```python
from build123d import *

# Parameters (mm, degrees)
CROQUIS2_R            = 43
CORTAR_EXTRUIR1_DEPTH = 2
CROQUIS4_R            = 40
CORTAR_EXTRUIR2_DEPTH = 3
CROQUIS6_R            = 30
CORTAR_EXTRUIR3_DEPTH = 8.5
CROQUIS8_R            = 30
CORTAR_EXTRUIR4_DEPTH = 1
CROQUIS9_R            = 25
CORTAR_EXTRUIR5_DEPTH = 1.5
CROQUIS10_R           = 15
CORTAR_EXTRUIR6_DEPTH = 13
CROQUIS11_R           = 12.5
CORTAR_EXTRUIR7_DEPTH = 18.5
CROQUIS12_R           = 9
CORTAR_EXTRUIR8_DEPTH = 22.5


with BuildPart() as part:
    # Croquis1 → Revolución1 (revolve)
    with BuildSketch(Plane.XY):
        Polygon((0, 0), (60, 0), (60, 12), (43, 12), (30, 27), (30, 35), (0, 35), align=None)
    revolve(axis=Axis((0, 35, 0), (0, -1, 0)))

    # Croquis2 → Cortar-Extruir1 (cut)
    with BuildSketch(Plane.XZ):
        Circle(CROQUIS2_R)
    extrude(amount=-CORTAR_EXTRUIR1_DEPTH, mode=Mode.SUBTRACT)

    # Croquis4 → Cortar-Extruir2 (cut)
    with BuildSketch(Plane.XZ.offset(-2)):
        Circle(CROQUIS4_R)
    extrude(amount=-CORTAR_EXTRUIR2_DEPTH, mode=Mode.SUBTRACT)

    # Croquis5 → Revolución2 (revolve)
    with BuildSketch(Plane.XY):
        Polygon((-40, 2), (-43, 0), (-43, 2), align=None)
    revolve(axis=Axis((0, 0, 0), (0, 1, 0)))

    # Croquis6 → Cortar-Extruir3 (cut)
    with BuildSketch(Plane.XZ.offset(-5)):
        Circle(CROQUIS6_R)
    extrude(amount=-CORTAR_EXTRUIR3_DEPTH, mode=Mode.SUBTRACT)

    # Croquis7 → Cortar-Revolución1 (revolve, cut)
    with BuildSketch(Plane.XY):
        Polygon((-40, 5), (-30, 5), (-30, 13.5), align=None)
    revolve(axis=Axis((0, 0, 0), (0, 1, 0)), mode=Mode.SUBTRACT)

    # Croquis8 → Cortar-Extruir4 (cut)
    with BuildSketch(Plane.XZ.offset(-13.5)):
        Circle(CROQUIS8_R)
    extrude(amount=-CORTAR_EXTRUIR4_DEPTH, mode=Mode.SUBTRACT)

    # Croquis9 → Cortar-Extruir5 (cut)
    with BuildSketch(Plane(origin=(0, 35, 0), x_dir=(1, 0, 0), z_dir=(0, 1, 0))):
        Circle(CROQUIS9_R)
    extrude(amount=-CORTAR_EXTRUIR5_DEPTH, mode=Mode.SUBTRACT)

    # Croquis10 → Cortar-Extruir6 (cut)
    with BuildSketch(Plane(origin=(0, 33.5, 0), x_dir=(1, 0, 0), z_dir=(0, 1, 0))):
        Circle(CROQUIS10_R)
    extrude(amount=-CORTAR_EXTRUIR6_DEPTH, mode=Mode.SUBTRACT)

    # Croquis11 → Cortar-Extruir7 (cut)
    with BuildSketch(Plane(origin=(0, 35, 0), x_dir=(1, 0, 0), z_dir=(0, 1, 0))):
        Circle(CROQUIS11_R)
    extrude(amount=-CORTAR_EXTRUIR7_DEPTH, mode=Mode.SUBTRACT)

    # Croquis12 → Cortar-Extruir8 (cut)
    with BuildSketch(Plane(origin=(0, 35, 0), x_dir=(1, 0, 0), z_dir=(0, 1, 0))):
        Circle(CROQUIS12_R)
    extrude(amount=-CORTAR_EXTRUIR8_DEPTH, mode=Mode.SUBTRACT)


solid = part.part
```
Verification items for the finished model (mm, model axes). A direction names the side the tool comes from. Round coordinates to 2 decimals unless told otherwise and drop trailing zeros. Write each loop counter-clockwise with the first axis right and the second up, starting at its lowest first coordinate (ties: lowest second). Pieces come first, ordered by that corner, then holes. Notation, with made-up numbers: (75.5, 22) - (94.5, 22) arc R17 cw to (94.5, 39) - close; hole circle Ø3 at (-26, 83.5). An arc over 180 degrees is marked (long way). Answer as a JSON object with one key per item and string values. Group by question number.
Q1. Tool access check on faces 4 (the cylindrical face through (-8.67, 3.48, -39.05)), 5 (the cylindrical face through (-1.172, 15.514, -8.923)), 6 (the cylindrical face through (-29.97, 31.06, 1.32)). Record the directions out of +Z, -Z, +X, -X, +Y, -Y that give a thin tool (end or side, any length) a straight path to the whole face; none if there is none.
Q2. Mould release check, pull along X, two halves, no side actions. Record for faces 1 (the flat face through (-14, 12, 41)), 2 (the cylindrical face through (-59.94, 6.08, 2.64)), 3 (the cylindrical face through (23.846, 34.26, -7.509)): released by +X, released by -X, zero draft, split by the parting line, or undercut.
Q3. Thickness scan on line 1 (X direction, y = 15.45, z = 0); line 2 (Z direction, x = 0, y = 2.85); line 3 (Y direction, x = -8.5, z = -13). Record the ranges inside material, lowest first.
Q4. Section check B-B, the plane y = 18.5. Enter the section's corners in (x, z).
Q5. Section check A-A, the plane y = 10. Enter the section's corners in (x, z), plus the area to 3 significant figures.
Q6. Go/stop test with flat-tipped pins: pin 1 Ø4 at (y, z) = (17.5, -5.5) entering from -X; pin 2 Ø4 at (y, z) = (5, 38) entering from -X; pin 3 Ø4 at (x, y) = (7.5, 15) entering from -Z. Record where each tip stops, or that it passes through.
Found:
{
 "1": {"face 4": "-Y", "face 5": "+Y, -Y", "face 6": "+Y"},
 "2": {"face 1": "zero draft", "face 2": "split by the parting line", "face 3": "undercut"},
 "3": {"line 1": "x = -40.01 to -9, 9 to 40.01", "line 2": "z = -60 to -40, 40 to 60", "line 3": "y = 14.5 to 33.5"},
 "4": {"outline": "circle Ø74.73 at (0, 0); hole circle Ø25 at (0, 0)"},
 "5": {"outline": "circle Ø120 at (0, 0); hole circle Ø68.24 at (0, 0)", "area": "7,650 mm^2"},
 "6": {"pin 1": "stops at x = -39.61", "pin 2": "stops at x = -48", "pin 3": "stops at z = -41.5"}
}
